```python
from build123d import *

# Parameters (mm, degrees)
SKETCH2_W               = 57
SKETCH2_H               = 141
BOSS_EXTRUDE1_DEPTH     = 20
SKETCH3_R               = 1.5
BOSS_EXTRUDE3_DEPTH     = 1
BOSS_EXTRUDE3_2_DEPTH   = 1
BOSS_EXTRUDE3_3_DEPTH   = 1
SKETCH4_W               = 43
SKETCH4_H               = 20
BOSS_EXTRUDE4_DEPTH     = 10
MIRROR1_START           = 19
MIRROR1_OUTLINE_R       = 1.5
MIRROR1_DEPTH           = 1
SHELL3_START            = -27.5
SHELL3_OUTLINE_W        = 19
SHELL3_OUTLINE_H        = 139
SHELL3_DEPTH            = 55
SHELL3_START_2          = 27.5
SHELL3_2_OUTLINE_W      = 19
SHELL3_2_OUTLINE_H      = 41
SHELL3_2_DEPTH          = 10
SKETCH10_R              = 1.5
BOSS_EXTRUDE5_DEPTH     = 1
MIRROR2_OUTLINE_W       = 1
MIRROR2_OUTLINE_H       = 41
MIRROR2_DEPTH           = 20
MIRROR2_2_DEPTH         = 1
MIRROR2_START           = 19
MIRROR2_3_OUTLINE_R     = 1.5
MIRROR2_3_DEPTH         = 1
SKETCH17_W              = 98
SKETCH17_H              = 20
BOSS_EXTRUDE7_DEPTH     = 2
CUT_EXTRUDE1_DEPTH      = 87.297450716
CUT_EXTRUDE1_DEPTH_BACK = 87.297450716
SKETCH11_W              = 45.81490068
SKETCH11_H              = 58.670112651
SKETCH13_W              = 18.731668524
SKETCH13_H              = 41
CUT_EXTRUDE15_DEPTH     = 87.297450716
SKETCH14_W              = 19.5
SKETCH14_H              = 13
CUT_EXTRUDE16_DEPTH     = 2
SKETCH15_R              = 1.5
BOSS_EXTRUDE6_DEPTH     = 1
SKETCH18_W              = 1
SKETCH18_H              = 19
BOSS_EXTRUDE8_DEPTH     = 1


# Read off the part's stored shape, not the designer's step: Mirror1, Shell3, Mirror2
with BuildPart() as part:
    # Sketch2 → Boss-Extrude1 (new body)
    with BuildSketch(Plane(origin=(0, 0, 0), x_dir=(1, 0, 0), z_dir=(0, 1, 0))):
        Rectangle(SKETCH2_W, SKETCH2_H)
    extrude(amount=BOSS_EXTRUDE1_DEPTH)

    # Sketch4 → Boss-Extrude4 (add)
    with BuildSketch(Plane(origin=(28.5, 0, 0), x_dir=(0, 0, -1), z_dir=(1, 0, 0))):
        with Locations((-49, 10)):
            Rectangle(SKETCH4_W, SKETCH4_H)
    extrude(amount=BOSS_EXTRUDE4_DEPTH)

    # Mirror1 outline → Mirror1 (add)
    with BuildSketch(Plane(origin=(0, 0, 0), x_dir=(1, 0, 0), z_dir=(0, 1, 0)).offset(MIRROR1_START)):
        with BuildLine():
            ThreePointArc((43.5, -67.652604127), (46, -65.152604127), (43.5, -62.652604127))
            Line((43.5, -62.652604127), (38.5, -62.652604127))
            Line((38.5, -62.652604127), (38.5, -67.652604127))
            Line((38.5, -67.652604127), (43.5, -67.652604127))
        make_face()
        with Locations((43.5, -65.152604127)):
            Circle(MIRROR1_OUTLINE_R, mode=Mode.SUBTRACT)
    extrude(amount=MIRROR1_DEPTH)

    # Shell3 outline → Shell3 (cut)
    with BuildSketch(Plane.YZ.offset(SHELL3_START)):
        with Locations((10.5, 0)):
            Rectangle(SHELL3_OUTLINE_W, SHELL3_OUTLINE_H)
    extrude(amount=SHELL3_DEPTH, mode=Mode.SUBTRACT)

    # Shell3 2 outline → Shell3 2 (cut)
    with BuildSketch(Plane.YZ.offset(SHELL3_START_2)):
        with Locations((10.5, 49)):
            Rectangle(SHELL3_2_OUTLINE_W, SHELL3_2_OUTLINE_H)
    extrude(amount=SHELL3_2_DEPTH, mode=Mode.SUBTRACT)

    # Sketch10 → Boss-Extrude5 (add)
    with BuildSketch(Plane(origin=(0, 20, 0), x_dir=(1, 0, 0), z_dir=(0, 1, 0))):
        with BuildLine():
            Line((33.5, -15), (28.5, -15))
            Line((28.5, -15), (28.5, -20))
            Line((28.5, -20), (33.5, -20))
            ThreePointArc((33.5, -20), (36, -17.5), (33.5, -15))
        make_face()
        with Locations(Location((33.5, -17.5, 0), (0, 0, 270))):
            Circle(SKETCH10_R, mode=Mode.SUBTRACT)
    extrude(amount=-BOSS_EXTRUDE5_DEPTH)


with BuildPart() as body_2:
    # Sketch3 → Boss-Extrude3 (new body)
    with BuildSketch(Plane(origin=(0, 20, 0), x_dir=(1, 0, 0), z_dir=(0, 1, 0))):
        with BuildLine():
            Line((-33.5, 67.652604127), (-28.5, 67.652604127))
            Line((-28.5, 67.652604127), (-28.5, 62.652604127))
            Line((-28.5, 62.652604127), (-33.5, 62.652604127))
            ThreePointArc((-33.5, 62.652604127), (-36, 65.152604127), (-33.5, 67.652604127))
        make_face()
        with Locations(Location((-33.5, 65.152604127, 0), (0, 0, 270))):
            Circle(SKETCH3_R, mode=Mode.SUBTRACT)
    extrude(amount=-BOSS_EXTRUDE3_DEPTH)



with BuildPart() as body_3:
    # Sketch3 → Boss-Extrude3 2 (new body)
    with BuildSketch(Plane(origin=(0, 20, 0), x_dir=(1, 0, 0), z_dir=(0, 1, 0))):
        with BuildLine():
            Line((-28.5, -67.652604127), (-28.5, -62.652604127))
            Line((-28.5, -62.652604127), (-33.5, -62.652604127))
            ThreePointArc((-33.5, -62.652604127), (-36, -65.152604127), (-33.5, -67.652604127))
            Line((-33.5, -67.652604127), (-28.5, -67.652604127))
        make_face()
        with Locations(Location((-33.5, -65.152604127, 0), (0, 0, 90))):
            Circle(SKETCH3_R, mode=Mode.SUBTRACT)
    extrude(amount=-BOSS_EXTRUDE3_2_DEPTH)


with BuildPart() as body_4:
    # Sketch3 → Boss-Extrude3 3 (new body)
    with BuildSketch(Plane(origin=(0, 20, 0), x_dir=(1, 0, 0), z_dir=(0, 1, 0))):
        with BuildLine():
            Line((28.5, 67.652604127), (28.5, 62.652604127))
            Line((28.5, 62.652604127), (33.5, 62.652604127))
            ThreePointArc((33.5, 62.652604127), (36, 65.152604127), (33.5, 67.652604127))
            Line((33.5, 67.652604127), (28.5, 67.652604127))
        make_face()
        with Locations(Location((33.5, 65.152604127, 0), (0, 0, 90))):
            Circle(SKETCH3_R, mode=Mode.SUBTRACT)
    extrude(amount=-BOSS_EXTRUDE3_3_DEPTH)


with BuildPart() as body_2_1:
    add(body_2.part)

    add(body_4.part)  # Mirror2 merges body 4

    add(part.part)  # Mirror2 merges part
    # Mirror2 outline → Mirror2 (add)
    with BuildSketch(Plane(origin=(0, 0, 0), x_dir=(1, 0, 0), z_dir=(0, 1, 0))):
        with Locations((28, -49)):
            Rectangle(MIRROR2_OUTLINE_W, MIRROR2_OUTLINE_H)
        Polygon((-28.5, -70.5), (-28.5, -69.5), (-37.5, -69.5), (-37.5, -28.5), (-28.5, -28.5), (-28.5, -27.5), (-38.5, -27.5), (-38.5, -70.5), align=None)
    extrude(amount=MIRROR2_DEPTH)

    # Mirror2 2 outline → Mirror2 2 (add)
    with BuildSketch(Plane(origin=(0, 0, 0), x_dir=(1, 0, 0), z_dir=(0, 1, 0))):
        Polygon((-37.5, -69.5), (-28.5, -69.5), (-28.5, -67.652604127), (-28.5, -62.652604127), (-28.5, -28.5), (-37.5, -28.5), align=None)
    extrude(amount=MIRROR2_2_DEPTH)

    # Mirror2 3 outline → Mirror2 3 (add)
    # profile 1 of 2: a face of its own
    with BuildSketch(Plane(origin=(0, 0, 0), x_dir=(1, 0, 0), z_dir=(0, 1, 0)).offset(MIRROR2_START)):
        with BuildLine():
            Line((-33.5, -20), (-28.5, -20))
            Line((-28.5, -20), (-28.5, -15))
            Line((-28.5, -15), (-33.5, -15))
            ThreePointArc((-33.5, -15), (-36, -17.5), (-33.5, -20))
        make_face()
        with Locations((-33.5, -17.5)):
            Circle(MIRROR2_3_OUTLINE_R, mode=Mode.SUBTRACT)
    # profile 2 of 2: a face of its own
    with BuildSketch(Plane(origin=(0, 0, 0), x_dir=(1, 0, 0), z_dir=(0, 1, 0)).offset(MIRROR2_START)):
        with BuildLine():
            Line((-43.5, -67.652604127), (-38.5, -67.652604127))
            Line((-38.5, -67.652604127), (-38.5, -62.652604127))
            Line((-38.5, -62.652604127), (-43.5, -62.652604127))
            ThreePointArc((-43.5, -62.652604127), (-46, -65.152604127), (-43.5, -67.652604127))
        make_face()
        with Locations((-43.5, -65.152604127)):
            Circle(MIRROR2_3_OUTLINE_R, mode=Mode.SUBTRACT)
    extrude(amount=MIRROR2_3_DEPTH)

    # Sketch17 → Boss-Extrude7 (add)
    with BuildSketch(Plane.ZY.offset(28.5)):
        with Locations((-21.5, 10)):
            Rectangle(SKETCH17_W, SKETCH17_H)
    extrude(amount=-BOSS_EXTRUDE7_DEPTH)

    # Sketch11 → Cut-Extrude1 (cut, two sides: drawn at the far end of the back side and taken through both)
    with BuildSketch(Plane(origin=(0, 1, 0), x_dir=(1, 0, 0), z_dir=(0, 1, 0)).offset(-CUT_EXTRUDE1_DEPTH_BACK)):
        with Locations((51.40745034, -56.835056326)):
            Rectangle(SKETCH11_W, SKETCH11_H)
    extrude(amount=CUT_EXTRUDE1_DEPTH + CUT_EXTRUDE1_DEPTH_BACK, mode=Mode.SUBTRACT)


with BuildPart() as cut_extrude15_tool:
    # Sketch13 → Cut-Extrude15 (new, through all)
    with BuildSketch(Plane(origin=(0, 1, 0), x_dir=(1, 0, 0), z_dir=(0, 1, 0))):
        with Locations((-28.134165738, -49)):
            Rectangle(SKETCH13_W, SKETCH13_H)
    extrude(amount=CUT_EXTRUDE15_DEPTH)


with BuildPart() as body_2_2:
    add(body_2_1.part)

    # Cut-Extrude15: cut by cut_extrude15_tool
    add(cut_extrude15_tool.part, mode=Mode.SUBTRACT)

    # Sketch14 → Cut-Extrude16 (cut)
    with BuildSketch(Plane.ZY.offset(28.5)):
        with Locations((-39.826302064, 10)):
            Rectangle(SKETCH14_W, SKETCH14_H)
        with Locations((-8.326302064, 10.017547542)):
            Rectangle(SKETCH14_W, SKETCH14_H)
    extrude(amount=-CUT_EXTRUDE16_DEPTH, mode=Mode.SUBTRACT)

    # Sketch15 → Boss-Extrude6 (add)
    with BuildSketch(Plane(origin=(0, 20, 0), x_dir=(1, 0, 0), z_dir=(0, 1, 0))):
        with BuildLine():
            Line((28.5, -67.652604127), (33.5, -67.652604127))
            ThreePointArc((33.5, -67.652604127), (36, -65.152604127), (33.5, -62.652604127))
            Line((33.5, -62.652604127), (28.5, -62.652604127))
            Line((28.5, -62.652604127), (28.5, -67.652604127))
        make_face()
        with Locations(Location((33.5, -65.152604127, 0), (0, 0, 90))):
            Circle(SKETCH15_R, mode=Mode.SUBTRACT)
    extrude(amount=-BOSS_EXTRUDE6_DEPTH)

    # Sketch18 → Boss-Extrude8 (add)
    with BuildSketch(Plane(origin=(-27.5, 0, 0), x_dir=(0, 0, -1), z_dir=(1, 0, 0))):
        with Locations((-28, 10.5)):
            Rectangle(SKETCH18_W, SKETCH18_H)
    extrude(amount=BOSS_EXTRUDE8_DEPTH)


with BuildPart() as body_3_1:
    add(body_3.part)

    # Cut-Extrude15: cut by cut_extrude15_tool
    add(cut_extrude15_tool.part, mode=Mode.SUBTRACT)


solid = body_2_2.part
```
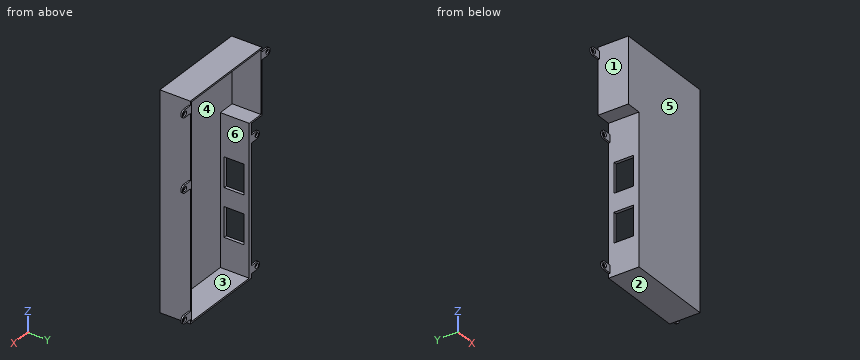
Work out the finished part from the listing and answer in its coordinate system (mm). Face numbers are marked on the shaded views. A direction names the side the tool comes from. Coordinates: 2 decimals unless noted, no trailing zeros. Loops run counter-clockwise (first coordinate to the right, second up) from the corner with the lowest first, then second, coordinate; pieces in that order, holes last. Notation, with made-up numbers: M 0.5,22 L 39.5,22 A33 cw 39.5,50 Z; hole C -4,-11 d3. An arc over 180 degrees is marked long. Use CSV: the item, a comma, the result in double quotes. Start each with the question number.
(1) Find section C-C, the plane x = -22.5. Give the vertices of the cut face in (y, z).
(2) Consider line 1 (X direction, y = 19.3, z = 17.5); line 2 (Z direction, x = -18.5, y = 9.5); line 3 (X direction, y = 2, z = 34). Determine where each line is inside the solid, lowest interval first.
(3) For the marked faces 5 and 6, determine the directions among +Z, -Z, +X, -X, +Y, -Y from which every point of the face is accessible in a straight line to the end or side of a thin tool.
(4) For a pull along Z with two mould halves and no side action, classify the marked faces 1, 2, 3 and 4 as +Z half, -Z half, draft (parallel to the pull), parting line (faces both ways), or undercut.
(5) Find section A-A, the plane z = -11.5. Give the vertices of the cut face in (x, y).
(6) Given pin 1 Ø5 at (y, z) = (17, 5.5) entering from -X; pin 2 Ø8 at (y, z) = (7.5, -7.5) entering from +X; pin 3 Ø2 at (x, z) = (-27.5, -38) entering from -Y; pin 4 Ø2 at (x, z) = (22, -31.5) entering from +Y, each flat-ended and moving along its own axis, determine where each tip first touches the part or whether it passes through.
(7) Find section D-D, the plane z = 49.5. Give the vertices of the cut face in (x, y), then the cut area to 3 significant figures.
(8) Find section B-B, the plane z = 17.5. Give the vertices of the cut face in (x, y).
Recorded:
1,outline,"M 0,-70.5 L 20,-70.5 L 20,-69.5 L 1,-69.5 L 1,69.5 L 20,69.5 L 20,70.5 L 0,70.5 Z"
2,line 1,"x = -36 to -35, -32 to -26.5, 27.5 to 32, 35 to 36"
2,line 2,"z = -70.5 to -69.5, 69.5 to 70.5"
2,line 3,"x = -38.5 to -37.5, 27.5 to 28.5"
3,face 5,"+Z, -Z, +X, -X, -Y"
3,face 6,"+Y"
4,face 1,"draft"
4,face 2,"-Z half"
4,face 3,"undercut"
4,face 4,"undercut"
5,outline,"M -28.5,0 L 28.5,0 L 28.5,20 L 27.5,20 L 27.5,1 L -26.5,1 L -26.5,3.52 L -28.5,3.52 Z; M -28.5,16.52 L -26.5,16.52 L -26.5,20 L -28.5,20 Z"
6,pin 1,"stops at x = -28.5"
6,pin 2,"stops at x = 28.5"
6,pin 3,"stops at y = 0"
6,pin 4,"stops at y = 1"
7,outline,"M -38.5,0 L 28.5,0 L 28.5,20 L 27.5,20 L 27.5,1 L -37.5,1 L -37.5,20 L -38.5,20 Z"
7,area,"105 mm^2"
8,outline,"M -36,19 L -35,19 L -35,20 L -36,20 Z; M -32,19 L -28.5,19 L -28.5,0 L 28.5,0 L 28.5,19 L 32,19 L 32,20 L 27.5,20 L 27.5,1 L -26.5,1 L -26.5,20 L -32,20 Z; M 35,19 L 36,19 L 36,20 L 35,20 Z"
